from build123d import *

# Parameters (mm, degrees)
SKETCH1_R               = 50.8
BOSS_EXTRUDE1_DEPTH     = 38.1
CUT_EXTRUDE_THIN2_START = -12.7
SKETCH22_R              = 50.8
SKETCH22_R_2            = 47.625
CUT_EXTRUDE_THIN2_DEPTH = 12.7
SKETCH24_R              = 57.15
BOSS_EXTRUDE3_DEPTH     = 6.35
CUT_EXTRUDE5_DEPTH      = 90.352420225
CUT_EXTRUDE5_DEPTH_BACK = 90.352420225
SKETCH20_R              = 8.9296875


with BuildPart() as part:
    # Sketch1 → Boss-Extrude1 (new body)
    with BuildSketch(Plane.XY):
        with Locations(Location((0, 0, 0), (0, 0, 180))):
            Circle(SKETCH1_R)
    extrude(amount=BOSS_EXTRUDE1_DEPTH)

    # Sketch22 → Cut-Extrude-Thin2 (cut)
    with BuildSketch(Plane.XY.offset(38.1).offset(CUT_EXTRUDE_THIN2_START)):
        Circle(SKETCH22_R)
        Circle(SKETCH22_R_2, mode=Mode.SUBTRACT)
    extrude(amount=CUT_EXTRUDE_THIN2_DEPTH, mode=Mode.SUBTRACT)

    # Sketch24 → Boss-Extrude3 (add)
    with BuildSketch(Plane.XY.offset(25.4)):
        Circle(SKETCH24_R)
    extrude(amount=-BOSS_EXTRUDE3_DEPTH)

    # Sketch20 → Cut-Extrude5 (cut, two sides: drawn at the far end of the back side and taken through both)
    with BuildSketch(Plane(origin=(0, 0, 0), x_dir=(-1, 0, 0), z_dir=(0, 0, -1)).offset(-CUT_EXTRUDE5_DEPTH_BACK)):
        with Locations((0, 19.05)):
            Circle(SKETCH20_R)
    extrude(amount=CUT_EXTRUDE5_DEPTH + CUT_EXTRUDE5_DEPTH_BACK, mode=Mode.SUBTRACT)


solid = part.part
Source: CAD feature listing. Evaluate the final solid. Frame: model axes, mm. A direction names the side the tool comes from. Coordinates: 2 decimals unless noted, no trailing zeros. Loops run counter-clockwise (first coordinate to the right, second up) from the corner with the lowest first, then second, coordinate; pieces in that order, holes last. Notation, with made-up numbers: (-1.75, -29.75) -> (52.25, -29.75) arc R34 cw to (52.25, 1.25) -> close; hole circle Ø9 at (-10.75, -36.75). An arc over 180 degrees is marked (long way). Answer in a Markdown table with one row per item. Add a question column.
Q1. Contact query for flat-ended pins moving along their axis: pin 1 Ø8 at (y, z) = (-32, 26) entering from +X; pin 2 Ø4 at (y, z) = (-25.5, 28.5) entering from -X; pin 3 Ø5 at (x, z) = (18, 13) entering from -Y; pin 4 Ø10.5 at (x, y) = (0, 19.05) entering from -Z. Output: stop coordinate, or through.
Q2. Ray query, line 1 along Y through (x, z) = (0, 10.5); line 2 along Y through (x, z) = (0, 26) (3 decimals); line 3 along Z through (x, y) = (46, -28). Return the intervals inside material, ascending.
Q3. Pull-direction query (Y, two-part tool) for faces 1 (the face through (1.2, 27.9, 19.3)), 2 (the face through (-57.095, 2.513, 22.269)), 3 (the face through (1, -1, 0)); classes: pulls with the +Y half, pulls with the -Y half, needs draft (parallel to the pull), parting line crosses it, or undercut.
Q4. Section A-A on x = 0. Return the cut outline in (y, z) (3 decimals), and give its area (3 significant figures).
Q5. Section C-C on y = 0. Return the cut outline in (x, z) (3 decimals).
Q6. Section B-B on y = 19.05. Return the cut outline in (x, z), and give its area (3 significant figures).
Q7. Reachability of faces 4 (the face through (-38, -34, 19.05)), 5 (the face through (1, -1, 38.1)), 6 (the face through (-37.794, -28.979, 31.661)) from +Z, -Z, +X, -X, +Y, -Y: full face, straight path, thin tool, end or side. Return the list, or none.
Q8. Section D-D on z = 21.5. Return the cut outline in (x, y), and give its area (3 significant figures).
Computed values:
| question | item | result |
|---|---|---|
| 1 | pin 1 | stops at x = 49.8 |
| 1 | pin 2 | stops at x = -41.42 |
| 1 | pin 3 | stops at y = -48.38 |
| 1 | pin 4 | passes through |
| 2 | line 1 | y = -50.8 to 10.12, 27.98 to 50.8 |
| 2 | line 2 | y = -47.625 to 10.12, 27.98 to 47.625 |
| 2 | line 3 | z = 19.05 to 25.4 |
| 3 | face 1 | undercut |
| 3 | face 2 | parting line crosses it |
| 3 | face 3 | needs draft |
| 4 | outline | (-57.15, 19.05) -> (-50.8, 19.05) -> (-50.8, 0) -> (10.12, 0) -> (10.12, 38.1) -> (-47.625, 38.1) -> (-47.625, 25.4) -> (-57.15, 25.4) -> close; (27.98, 0) -> (50.8, 0) -> (50.8, 19.05) -> (57.15, 19.05) -> (57.15, 25.4) -> (47.625, 25.4) -> (47.625, 38.1) -> (27.98, 38.1) -> close |
| 4 | area | 3,190 mm^2 |
| 5 | outline | (-57.15, 19.05) -> (-50.8, 19.05) -> (-50.8, 0) -> (50.8, 0) -> (50.8, 19.05) -> (57.15, 19.05) -> (57.15, 25.4) -> (47.625, 25.4) -> (47.625, 38.1) -> (-47.625, 38.1) -> (-47.625, 25.4) -> (-57.15, 25.4) -> close |
| 6 | outline | (-53.88, 19.05) -> (-47.09, 19.05) -> (-47.09, 0) -> (-8.93, 0) -> (-8.93, 38.1) -> (-43.65, 38.1) -> (-43.65, 25.4) -> (-53.88, 25.4) -> close; (8.93, 0) -> (47.09, 0) -> (47.09, 19.05) -> (53.88, 19.05) -> (53.88, 25.4) -> (43.65, 25.4) -> (43.65, 38.1) -> (8.93, 38.1) -> close |
| 6 | area | 2,910 mm^2 |
| 7 | face 4 | -Z |
| 7 | face 5 | +Z, +X, -X, +Y, -Y |
| 7 | face 6 | +Z |
| 8 | outline | circle Ø114.3 at (0, 0); hole circle Ø17.86 at (0, 19.05) |
| 8 | area | 10,000 mm^2 |
